from build123d import *

# Parameters (mm, degrees)
SKETCH1_W           = 129.6416
SKETCH1_H           = 31.75
SKETCH1_R           = 2.1336
SKETCH1_R_2         = 5.588
SKETCH1_R_3         = 1.4732
BOSS_EXTRUDE1_DEPTH = 0.4064
FILLET1_R           = 0.381


with BuildPart() as part:
    # Sketch1 → Boss-Extrude1 (new body)
    with BuildSketch(Plane.XY):
        Rectangle(SKETCH1_W, SKETCH1_H)
        with Locations((58.7248, 9.525)):
            Circle(SKETCH1_R, mode=Mode.SUBTRACT)
        with Locations((58.7248, -9.525)):
            Circle(SKETCH1_R, mode=Mode.SUBTRACT)
        Circle(SKETCH1_R_2, mode=Mode.SUBTRACT)
        with Locations((0, 9.525)):
            Circle(SKETCH1_R_3, mode=Mode.SUBTRACT)
        with Locations((0, -9.525)):
            Circle(SKETCH1_R_3, mode=Mode.SUBTRACT)
        with Locations((-58.7248, 9.525)):
            Circle(SKETCH1_R, mode=Mode.SUBTRACT)
        with Locations((-58.7248, -9.525)):
            Circle(SKETCH1_R, mode=Mode.SUBTRACT)
    extrude(amount=BOSS_EXTRUDE1_DEPTH)

    # Fillet1
    fillet1_edges = [part.edges().sort_by_distance(p)[0] for p in [
        (-64.8208, 15.875, 0.2032),
        (64.8208, 15.875, 0.2032),
        (64.8208, -15.875, 0.2032),
        (-64.8208, -15.875, 0.2032),
    ]]
    fillet(fillet1_edges, radius=FILLET1_R)


solid = part.part
The model under review builds one solid part; all positions refer to its coordinate system, in mm. Round coordinates to 2 decimals unless told otherwise and drop trailing zeros. Order: outer loops, then holes, each group sorted by start corner. A loop starts at its lowest first (then second) coordinate and runs counter-clockwise, first axis right, second up. Notation, with made-up numbers: (84, -5.5) -> (124, -5.5) arc R18 ccw to (124, 20.5) -> close; hole circle Ø2 at (28.25, 31). An arc over 180 degrees is marked (long way). Write item = value, one per line. Start each with the question number.
Item 1: For line 1 along Y through (x, z) = (0, 0.2) (3 decimals); line 2 along X through (y, z) = (-10.5, 0.1); line 3 along Y through (x, z) = (57.5, 0.2) (3 decimals), list the stretches that pass through material, from the lowest coordinate up.
Item 2: Mouldability with a two-part tool opening along X and no side actions: class faces 1 (the face through (-1, 7, 0.406)), 2 (the face through (0.68, 8.22, 0.2)), 3 (the face through (60.76, 10.17, 0.2)) as released by +X, released by -X, zero draft, split by the parting line, or undercut.
Item 3: Consider section B-B on y = 0. Write out the cut boundary in (x, z), plus the area to 3 significant figures.
Item 4: Consider section A-A on x = 0. Write out the cut boundary in (y, z) (3 decimals), plus the area to 3 significant figures.
Item 5: Consider section C-C on z = 0.25. Write out the cut boundary in (x, y) (3 decimals), plus the area to 3 significant figures.
Conclusion:
q1.line_1 = -15.875 to -10.998, -8.052 to -5.588, 5.588 to 8.052, 10.998 to 15.875
q1.line_2 = -64.82 to -60.62, -56.83 to -1.1, 1.1 to 56.83, 60.62 to 64.82
q1.line_3 = -15.875 to -11.272, -7.778 to 7.778, 11.272 to 15.875
q2.face_1 = zero draft
q2.face_2 = undercut
q2.face_3 = undercut
q3.outline = (-64.82, 0) -> (-5.59, 0) -> (-5.59, 0.41) -> (-64.82, 0.41) -> close; (5.59, 0) -> (64.82, 0) -> (64.82, 0.41) -> (5.59, 0.41) -> close
q3.area = 48.1 mm2
q4.outline = (-15.875, 0) -> (-10.998, 0) -> (-10.998, 0.406) -> (-15.875, 0.406) -> close; (-8.052, 0) -> (-5.588, 0) -> (-5.588, 0.406) -> (-8.052, 0.406) -> close; (5.588, 0) -> (8.052, 0) -> (8.052, 0.406) -> (5.588, 0.406) -> close; (10.998, 0) -> (15.875, 0) -> (15.875, 0.406) -> (10.998, 0.406) -> close
q4.area = 5.97 mm2
q5.outline = (-64.821, -15.494) arc R0.381 ccw to (-64.44, -15.875) -> (64.44, -15.875) arc R0.381 ccw to (64.821, -15.494) -> (64.821, 15.494) arc R0.381 ccw to (64.44, 15.875) -> (-64.44, 15.875) arc R0.381 ccw to (-64.821, 15.494) -> close; hole circle Ø4.267 at (-58.725, -9.525); hole circle Ø4.267 at (-58.725, 9.525); hole circle Ø11.176 at (0, 0); hole circle Ø2.946 at (0, -9.525); hole circle Ø2.946 at (0, 9.525); hole circle Ø4.267 at (58.725, -9.525); hole circle Ø4.267 at (58.725, 9.525)
q5.area = 3,950 mm2
